Check sheet for the drawn part. Datum: minimum x, y, z corner. Units: mm. Round coordinates to 2 decimals unless told otherwise and drop trailing zeros. Write each loop counter-clockwise with the first axis right and the second up, starting at its lowest first coordinate (ties: lowest second). Pieces come first, ordered by that corner, then holes.
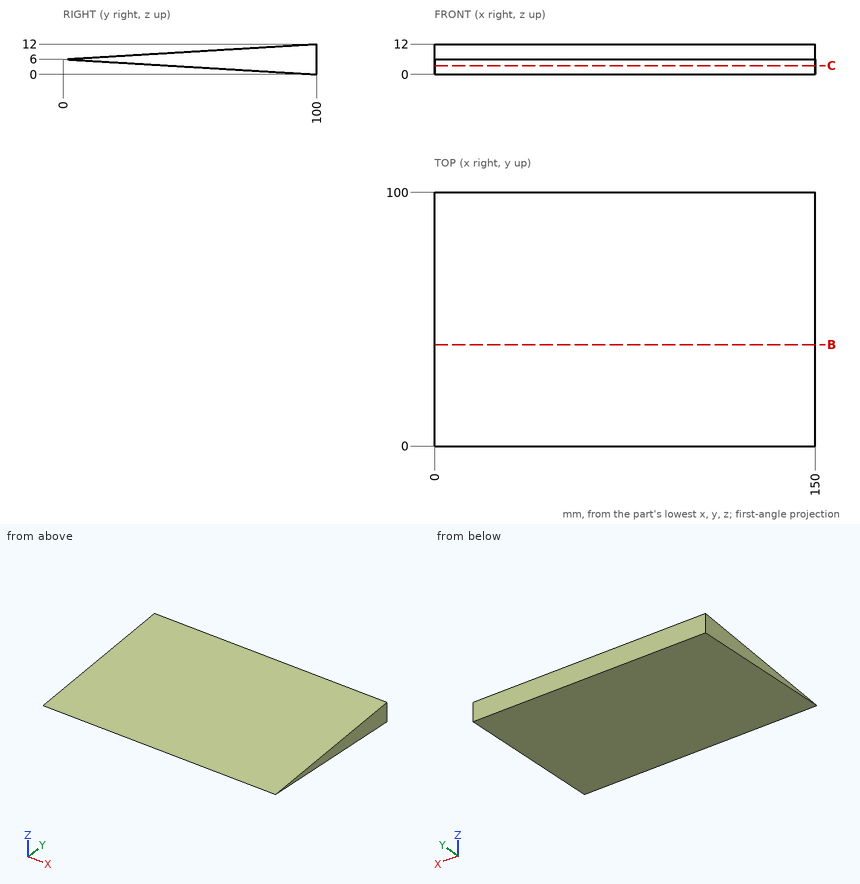
1. Sectioned sample at B-B, the plane y = 40. Enter the section's corners in (x, z), plus the area to 3 significant figures.
2. Scan lines: line 1 along Z through (x, y) = (110.5, 42); line 2 along Z through (x, y) = (44, 9). Record each from-to range of solid material in increasing order.
3. Go/stop test with flat-tipped pins: pin 1 (6 mm diameter, centred on x = 20, y = 29.5, fed in from +Z); pin 2 (5 mm diameter, centred on x = 110.5, y = 42, fed in from -Z); pin 3 (4 mm diameter, centred on x = 21.5, y = 35.5, fed in from +Z); pin 4 (6 mm diameter, centred on y = 36, z = 11, fed in from +X). Record where each tip stops, or that it passes through.
4. Sectioned sample at C-C, the plane z = 3.5. Enter the section's corners in (x, y), plus the area to 3 significant figures.
Computed values:
1. outline: (0, 3.6) - (150, 3.6) - (150, 8.4) - (0, 8.4) - close
1. area: 720 mm2
2. line 1: z = 3.48 to 8.52
2. line 2: z = 5.46 to 6.54
3. pin 1: stops at z = 7.95
3. pin 2: stops at z = 3.33
3. pin 3: stops at z = 8.25
3. pin 4: stops at x = 150
4. outline: (0, 41.67) - (150, 41.67) - (150, 100) - (0, 100) - close
4. area: 8,750 mm2
